Source: CAD feature listing. Evaluate the final solid. Frame: model axes, mm. A direction names the side the tool comes from. Coordinates: 2 decimals unless noted, no trailing zeros. Loops run counter-clockwise (first coordinate to the right, second up) from the corner with the lowest first, then second, coordinate; pieces in that order, holes last. Notation, with made-up numbers: (16, 56.5) - (59, 56.5) arc R19 ccw to (59, 60.5) - close; hole circle Ø5 at (-21.5, 22.25). An arc over 180 degrees is marked (long way). Write item = value, one per line. Start each with the question number.
from build123d import *

# Parameters (mm, degrees)
SKETCH1_R           = 4.75
BOSS_EXTRUDE1_DEPTH = 11
CUT_EXTRUDE1_DEPTH  = 1
CUT_EXTRUDE2_START  = -1
CUT_EXTRUDE2_DEPTH  = 1


with BuildPart() as part:
    # Sketch1 → Boss-Extrude1 (new body)
    with BuildSketch(Plane(origin=(0, 0, 0), x_dir=(1, 0, 0), z_dir=(0, 1, 0))):
        with BuildLine():
            Line((19.491292084, 0.988927265), (41.991292084, -3.793595372))
            ThreePointArc((41.991292084, -3.793595372), (43.725917616, -4.524537322), (45.067363393, -5.845039159))
            ThreePointArc((45.067363393, -5.845039159), (50.669911309, -7.779535303), (54.182993157, -3.005744942))
            Line((54.182993157, -3.005744942), (54.182993157, 8.494255058))
            ThreePointArc((54.182993157, 8.494255058), (53.011420282, 11.322682182), (50.182993157, 12.494255058))
            Line((50.182993157, 12.494255058), (-37.817006843, 12.494255058))
            ThreePointArc((-37.817006843, 12.494255058), (-46.817006843, 3.494255058), (-37.817006843, -5.505744942))
            Line((-37.817006843, -5.505744942), (11.462947477, -5.505744942))
            ThreePointArc((11.462947477, -5.505744942), (12.836569821, -4.959416727), (13.459743521, -3.618906598))
            ThreePointArc((13.459743521, -3.618906598), (15.416365081, 0.071416888), (19.491292084, 0.988927265))
        make_face()
        with Locations(Location((-37.817006843, 3.494255058, 0), (0, 0, 270))):
            Circle(SKETCH1_R, mode=Mode.SUBTRACT)
    extrude(amount=BOSS_EXTRUDE1_DEPTH)

    # Sketch2 → Cut-Extrude1 (cut)
    with BuildSketch(Plane(origin=(0, 11, 0), x_dir=(1, 0, 0), z_dir=(0, 1, 0))):
        with BuildLine():
            Line((50.182993157, 11.494255058), (-37.817006843, 11.494255058))
            ThreePointArc((-37.817006843, 11.494255058), (-45.817006843, 3.494255058), (-37.817006843, -4.505744942))
            Line((-37.817006843, -4.505744942), (11.462947477, -4.505744942))
            ThreePointArc((11.462947477, -4.505744942), (12.149758649, -4.232580835), (12.461345499, -3.56232577))
            ThreePointArc((12.461345499, -3.56232577), (14.809291371, 0.866062414), (19.699203775, 1.967074866))
            Line((19.699203775, 1.967074866), (42.199203775, -2.815447772))
            ThreePointArc((42.199203775, -2.815447772), (44.280754414, -3.692578112), (45.890489346, -5.277180316))
            ThreePointArc((45.890489346, -5.277180316), (50.372527679, -6.824777231), (53.182993157, -3.005744942))
            Line((53.182993157, -3.005744942), (53.182993157, 8.494255058))
            ThreePointArc((53.182993157, 8.494255058), (52.3043135, 10.615575401), (50.182993157, 11.494255058))
        make_face()
    extrude(amount=-CUT_EXTRUDE1_DEPTH, mode=Mode.SUBTRACT)

    # Sketch3 → Cut-Extrude2 (cut)
    with BuildSketch(Plane.XZ.offset(CUT_EXTRUDE2_START)):
        with BuildLine():
            Line((11.462947477, 4.505744942), (-37.817006843, 4.505744942))
            ThreePointArc((-37.817006843, 4.505744942), (-45.817006843, -3.494255058), (-37.817006843, -11.494255058))
            Line((-37.817006843, -11.494255058), (50.182993157, -11.494255058))
            ThreePointArc((50.182993157, -11.494255058), (52.3043135, -10.615575401), (53.182993157, -8.494255058))
            Line((53.182993157, -8.494255058), (53.182993157, 3.005744942))
            ThreePointArc((53.182993157, 3.005744942), (50.372527679, 6.824777231), (45.890489346, 5.277180316))
            ThreePointArc((45.890489346, 5.277180316), (44.280754414, 3.692578112), (42.199203775, 2.815447772))
            Line((42.199203775, 2.815447772), (19.699203775, -1.967074866))
            ThreePointArc((19.699203775, -1.967074866), (14.809291371, -0.866062414), (12.461345499, 3.56232577))
            ThreePointArc((12.461345499, 3.56232577), (12.149758649, 4.232580835), (11.462947477, 4.505744942))
        make_face()
    extrude(amount=CUT_EXTRUDE2_DEPTH, mode=Mode.SUBTRACT)


solid = part.part
Item 1: Cut plane D-D (x = 21). Return the cut outline in (y, z).
Item 2: Cut plane B-B (x = 9.5). Return the cut outline in (y, z), then the cut area to 3 significant figures.
Item 3: First-contact query: pin 1 (3 mm diameter, centred on x = 39, y = 9.5, fed in from +Z); pin 2 (0.8 mm diameter, centred on y = 0.5, z = -5, fed in from -X); pin 3 (2 mm diameter, centred on y = 3, z = -10, fed in from +X); pin 4 (8.5 mm diameter, centred on x = -37.82, z = -3.49, fed in from +Y). Flat tips, straight axial feed; report the tip coordinate or a pass-through.
Item 4: Material intervals for L1, parallel to Y at x = -42, z = -6; L2, parallel to Z at x = 5, y = 9.75; L3, parallel to Z at x = -14.5, y = 10.5, sorted ascending. Write a range as [from, to].
Item 5: Cut plane C-C (z = -5). Return the cut outline in (x, y), then the cut area to 3 significant figures.
Item 6: Draft query along Z for faces 5 (the flat face through (3, 10, -4)), 6 (the cylindrical face through (15.369, 5.423, -0.035)), 7 (the cylindrical face through (44.31, 0.51, 3.71)), 8 (the cylindrical face through (-46.815, 5.423, -3.692)). Return one class per face: released by +Z, released by -Z, zero draft, split by the parting line, or undercut.
Item 7: Reachability of faces 1 (the flat face through (-14, 5, 5.506)), 2 (the cylindrical face through (52.28, 0.51, -10.64)), 3 (the cylindrical face through (12.821, 5.423, 4.974)), 4 (the cylindrical face through (44.25, 10.51, 3.67)) from +Z, -Z, +X, -X, +Y, -Y: full face, straight path, thin tool, end or side. Return the list, or none.
Item 8: Cut plane A-A (y = 4). Return the cut outline in (x, z), then the cut area to 3 significant figures.
Responses:
q1.outline = (0, -12.49) - (11, -12.49) - (11, -11.49) - (10, -11.49) - (10, -1.69) - (11, -1.69) - (11, -0.67) - (0, -0.67) - (0, -1.69) - (1, -1.69) - (1, -11.49) - (0, -11.49) - close
q2.outline = (0, -12.49) - (11, -12.49) - (11, -11.49) - (10, -11.49) - (10, 4.51) - (11, 4.51) - (11, 5.51) - (0, 5.51) - (0, 4.51) - (1, 4.51) - (1, -11.49) - (0, -11.49) - close
q2.area = 166 mm2
q3.pin_1 = 3.48
q3.pin_2 = -46.75
q3.pin_3 = 54.15
q3.pin_4 = through
q4.L1 = [1, 10]
q4.L2 = [-12.49, 5.51]
q4.L3 = [-12.49, -11.49], [4.51, 5.51]
q5.outline = (-46.69, 0) - (-45.67, 0) - (-45.67, 1) - (-42.32, 1) - (-42.32, 10) - (-45.67, 10) - (-45.67, 11) - (-46.69, 11) - close; (-33.31, 1) - (53.18, 1) - (53.18, 0) - (54.18, 0) - (54.18, 11) - (53.18, 11) - (53.18, 10) - (-33.31, 10) - close
q5.area = 831 mm2
q6.face_5 = undercut
q6.face_6 = released by +Z
q6.face_7 = undercut
q6.face_8 = split by the parting line
q7.face_1 = +Z, -X, +Y, -Y
q7.face_2 = -Y
q7.face_3 = +Z, +Y, -Y
q7.face_4 = +Y
q8.outline = (-37.82, -12.49) - (50.18, -12.49) arc R4 ccw to (54.18, -8.49) - (54.18, 3.01) arc R5 ccw to (45.07, 5.85) arc R5 cw to (41.99, 3.79) - (19.49, -0.99) arc R5 cw to (13.46, 3.62) arc R2 ccw to (11.46, 5.51) - (-37.82, 5.51) arc R9 ccw to start; hole circle Ø9.5 at (-37.82, -3.49)
q8.area = 1,590 mm2
